Geometry: final body of the model. Coordinates: model frame, mm. A direction names the side the tool comes from. Give positions to 0.01 mm unless a question says otherwise; leave off trailing zeros. Write each loop counter-clockwise with the first axis right and the second up, starting at its lowest first coordinate (ties: lowest second). Pieces come first, ordered by that corner, then holes.
```python
from build123d import *

# Parameters (mm, degrees)
SKETCH1_R           = 11
BOSS_EXTRUDE1_DEPTH = 3.7
CUT_EXTRUDE1_REACH  = 17.99
SKETCH2_R           = 1.5
BOSS_EXTRUDE2_START = 2
SKETCH3_R           = 5
BOSS_EXTRUDE2_DEPTH = 10.6
CUT_EXTRUDE2_REACH  = 20.824
SKETCH4_R           = 3.5


with BuildPart() as part:
    # Sketch1 → Boss-Extrude1 (new body)
    with BuildSketch(Plane(origin=(0, 0, 0), x_dir=(1, 0, 0), z_dir=(0, 1, 0))):
        with Locations(Location((0, 0, 0), (0, 0, 270))):
            Circle(SKETCH1_R)
    extrude(amount=BOSS_EXTRUDE1_DEPTH)

    # Sketch2 → Cut-Extrude1 (cut, up to next)
    with BuildSketch(Plane(origin=(0, 3.7, 0), x_dir=(1, 0, 0), z_dir=(0, 1, 0)), mode=Mode.PRIVATE) as cut_extrude1_sk1:
        with Locations(Location((0, 8, 0), (0, 0, 270))):
            Circle(SKETCH2_R)
    cut_extrude1_tool1 = extrude(cut_extrude1_sk1.sketch, amount=-CUT_EXTRUDE1_REACH, mode=Mode.PRIVATE) & part.part
    # Sketch2 → Cut-Extrude1 (cut, up to next)
    with BuildSketch(Plane(origin=(0, 3.7, 0), x_dir=(1, 0, 0), z_dir=(0, 1, 0)), mode=Mode.PRIVATE) as cut_extrude1_sk2:
        with Locations(Location((8, 0, 0), (0, 0, 270))):
            Circle(SKETCH2_R)
    cut_extrude1_tool2 = extrude(cut_extrude1_sk2.sketch, amount=-CUT_EXTRUDE1_REACH, mode=Mode.PRIVATE) & part.part
    # Sketch2 → Cut-Extrude1 (cut, up to next)
    with BuildSketch(Plane(origin=(0, 3.7, 0), x_dir=(1, 0, 0), z_dir=(0, 1, 0)), mode=Mode.PRIVATE) as cut_extrude1_sk3:
        with Locations(Location((0, -8, 0), (0, 0, 270))):
            Circle(SKETCH2_R)
    cut_extrude1_tool3 = extrude(cut_extrude1_sk3.sketch, amount=-CUT_EXTRUDE1_REACH, mode=Mode.PRIVATE) & part.part
    # Sketch2 → Cut-Extrude1 (cut, up to next)
    with BuildSketch(Plane(origin=(0, 3.7, 0), x_dir=(1, 0, 0), z_dir=(0, 1, 0)), mode=Mode.PRIVATE) as cut_extrude1_sk4:
        with Locations(Location((-8, 0, 0), (0, 0, 270))):
            Circle(SKETCH2_R)
    cut_extrude1_tool4 = extrude(cut_extrude1_sk4.sketch, amount=-CUT_EXTRUDE1_REACH, mode=Mode.PRIVATE) & part.part
    add(cut_extrude1_tool1.solids().sort_by_distance((0, 3.7, -8))[0], mode=Mode.SUBTRACT)
    add(cut_extrude1_tool2.solids().sort_by_distance((8, 3.7, 0))[0], mode=Mode.SUBTRACT)
    add(cut_extrude1_tool3.solids().sort_by_distance((0, 3.7, 8))[0], mode=Mode.SUBTRACT)
    add(cut_extrude1_tool4.solids().sort_by_distance((-8, 3.7, 0))[0], mode=Mode.SUBTRACT)

    # Sketch3 → Boss-Extrude2 (add)
    with BuildSketch(Plane(origin=(0, 3.7, 0), x_dir=(1, 0, 0), z_dir=(0, 1, 0)).offset(BOSS_EXTRUDE2_START)):
        with Locations(Location((0, 0, 0), (0, 0, 270))):
            Circle(SKETCH3_R)
    extrude(amount=-BOSS_EXTRUDE2_DEPTH)

    # Sketch4 → Cut-Extrude2 (cut, up to next)
    with BuildSketch(Plane(origin=(0, 5.7, 0), x_dir=(1, 0, 0), z_dir=(0, 1, 0)), mode=Mode.PRIVATE) as cut_extrude2_sk1:
        with Locations(Location((0, 0, 0), (0, 0, 270))):
            Circle(SKETCH4_R)
    cut_extrude2_tool1 = extrude(cut_extrude2_sk1.sketch, amount=-CUT_EXTRUDE2_REACH, mode=Mode.PRIVATE) & part.part
    add(cut_extrude2_tool1.solids().sort_by_distance((0, 5.7, 0))[0], mode=Mode.SUBTRACT)


solid = part.part
```
Item 1: Section C-C, the plane y = 0.75. Return the cut outline in (x, z).
Found:
outline: circle Ø22 at (0, 0); hole circle Ø3 at (-8, 0); hole circle Ø7 at (0, 0); hole circle Ø3 at (0, -8); hole circle Ø3 at (0, 8); hole circle Ø3 at (8, 0)
Item 2: Section A-A, the plane z = 0. Return the cut outline in (x, y).
Found:
outline: (-11, 0) - (-9.5, 0) - (-9.5, 3.7) - (-11, 3.7) - close; (-6.5, 0) - (-5, 0) - (-5, -4.9) - (-3.5, -4.9) - (-3.5, 5.7) - (-5, 5.7) - (-5, 3.7) - (-6.5, 3.7) - close; (3.5, -4.9) - (5, -4.9) - (5, 0) - (6.5, 0) - (6.5, 3.7) - (5, 3.7) - (5, 5.7) - (3.5, 5.7) - close; (9.5, 0) - (11, 0) - (11, 3.7) - (9.5, 3.7) - close
Item 3: Reachability of faces 5 (the face through (-5, 3.7, 2)), 6 (the face through (6.536, 1.876, -0.325)), 7 (the face through (-4.88, -2.42, -1.08)) from +Z, -Z, +X, -X, +Y, -Y: full face, straight path, thin tool, end or side. Return the list, or none.
Found:
face 5: +Y
face 6: +Y, -Y
face 7: -Y
Item 4: Section B-B, the plane x = 0. Return the cut outline in (y, z), plus the area to 3 significant figures.
Found:
outline: (-4.9, -5) - (0, -5) - (0, -6.5) - (3.7, -6.5) - (3.7, -5) - (5.7, -5) - (5.7, -3.5) - (-4.9, -3.5) - close; (-4.9, 3.5) - (5.7, 3.5) - (5.7, 5) - (3.7, 5) - (3.7, 6.5) - (0, 6.5) - (0, 5) - (-4.9, 5) - close; (0, -11) - (3.7, -11) - (3.7, -9.5) - (0, -9.5) - close; (0, 9.5) - (3.7, 9.5) - (3.7, 11) - (0, 11) - close
area: 54.0 mm2
Item 5: Pin query (flat end, axial travel): pin 1 Ø1 at (x, z) = (1.5, -7.5) entering from +Y; pin 2 Ø5 at (y, z) = (-1.5, -4.5) entering from -X; pin 3 Ø2 at (x, y) = (-4.5, 1.5) entering from +Z. Return the tip coordinate at first contact, or that it passes through.
Found:
pin 1: stops at y = 3.7
pin 2: stops at x = -10.71
pin 3: stops at z = 10.43
Item 6: Line query: L1, parallel to X at y = 0.95, z = 0; L2, parallel to Y at x = 5, z = -7.25; L3, parallel to X at y = 0.5, z = 7.25. Output: solid intervals per line, ascending.
Found:
L1: x = -11 to -9.5, -6.5 to -3.5, 3.5 to 6.5, 9.5 to 11
L2: y = 0 to 3.7
L3: x = -8.27 to -1.3, 1.3 to 8.27
Item 7: Section D-D, the plane z = 8. Return the cut outline in (x, y).
Found:
outline: (-7.55, 0) - (-1.5, 0) - (-1.5, 3.7) - (-7.55, 3.7) - close; (1.5, 0) - (7.55, 0) - (7.55, 3.7) - (1.5, 3.7) - close
Item 8: Pull-direction query (X, two-part tool) for faces 1 (the face through (-3.417, 0.474, -0.759)), 2 (the face through (-4.88, 4.71, -1.08)), 3 (the face through (-5, 0, 2)), 4 (the face through (0.07, 1.88, 6.5)); classes: +X half, -X half, draft (parallel to the pull), parting line (faces both ways), or undercut.
Found:
face 1: undercut
face 2: parting line
face 3: draft
face 4: undercut
